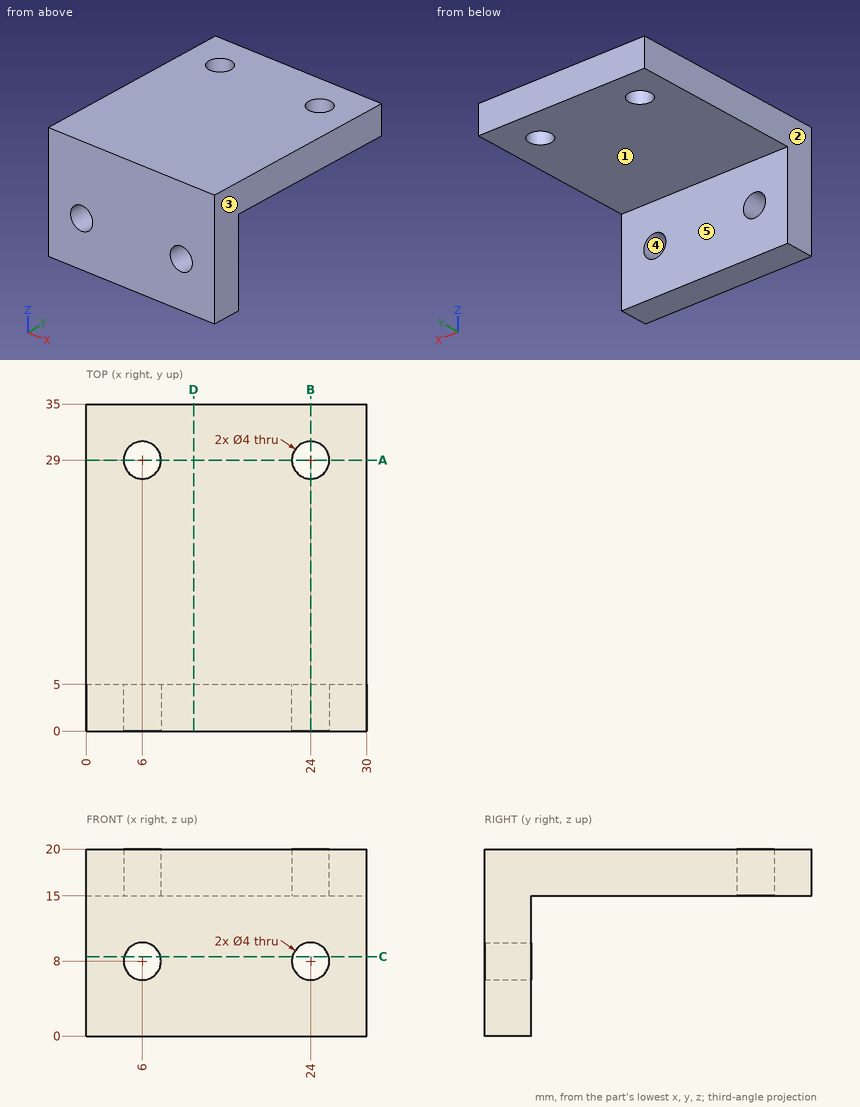
Answer from the drawing. Dimensions are ordinates in mm from the lowest x, y and z of the part. A direction names the side the tool comes from. Give positions to 0.01 mm unless a question says otherwise; leave off trailing zeros. Write each loop counter-clockwise with the first axis right and the second up, starting at its lowest first coordinate (ties: lowest second). Pieces come first, ordered by that corner, then holes.
1) Section D-D (x = 11.5) is taken. Write down the section's boundary in (y, z).
2) For a pull along X with two mould halves and no side action, classify the marked faces 3, 4 and 5 as pulls with the +X half, pulls with the -X half, needs draft (parallel to the pull), parting line crosses it, or undercut.
3) Section B-B (x = 24) is taken. Write down the section's boundary in (y, z).
4) Section A-A (y = 29) is taken. Write down the section's boundary in (x, z).
5) Section C-C (z = 8.5) is taken. Write down the section's boundary in (x, y), and give its area (3 significant figures).
6) Find the intervals of material crossed by L1, parallel to Y at x = 6, z = 17.75; L2, parallel to Z at x = 24, y = 3.5; L3, parallel to Y at x = 14.75, z = 14.75, in increasing order.
7) Given P1, Ø5, axis at x = 14.5, y = 17, coming from the -Z side; P2, Ø3.5, axis at x = 24, z = 8, coming from the +Y side; P3, Ø2, axis at x = 13.5, z = 4, coming from the +Y side, each flat-ended and moving along its own axis, determine where each tip first touches the part or whether it passes through.
8) A tool of negligible diameter and unlimited length cuts with its end or side. For the marked faces 1 and 2, from which of +Z, -Z, +X, -X, +Y, -Y can it reach the whole face along a straight path? Write none if from no direction.
Response:
1. outline: (0, 0) - (5, 0) - (5, 15) - (35, 15) - (35, 20) - (0, 20) - close
2. face 3: pulls with the +X half
2. face 4: undercut
2. face 5: needs draft
3. outline: (0, 0) - (5, 0) - (5, 6) - (0, 6) - close; (0, 10) - (5, 10) - (5, 15) - (27, 15) - (27, 20) - (0, 20) - close; (31, 15) - (35, 15) - (35, 20) - (31, 20) - close
4. outline: (0, 15) - (4, 15) - (4, 20) - (0, 20) - close; (8, 15) - (22, 15) - (22, 20) - (8, 20) - close; (26, 15) - (30, 15) - (30, 20) - (26, 20) - close
5. outline: (0, 0) - (4.06, 0) - (4.06, 5) - (0, 5) - close; (7.94, 0) - (22.06, 0) - (22.06, 5) - (7.94, 5) - close; (25.94, 0) - (30, 0) - (30, 5) - (25.94, 5) - close
5. area: 111 mm2
6. L1: y = 0 to 27, 31 to 35
6. L2: z = 0 to 6, 10 to 20
6. L3: y = 0 to 5
7. P1: stops at z = 15
7. P2: passes through
7. P3: stops at y = 5
8. face 1: -Z, +X, -X, +Y
8. face 2: +Z, -Z, -X, +Y, -Y
